```python
from build123d import *

# Parameters (mm, degrees)
BOSS_EXTRUDE1_DEPTH = 8
SKETCH2_R           = 5
BOSS_EXTRUDE2_DEPTH = 28
FILLET1_R           = 2
SKETCH3_R           = 1.55
CUT_EXTRUDE1_DEPTH  = 15.6
FILLET2_R           = 1
SKETCH5_R           = 2.1
CUT_EXTRUDE3_DEPTH  = 4
SKETCH6_R           = 0.5
CUT_EXTRUDE4_DEPTH  = 0.5
CUT_EXTRUDE5_REACH  = 10
SKETCH7_R           = 1


with BuildPart() as part:
    # Sketch1 → Boss-Extrude1 (new body)
    with BuildSketch(Plane(origin=(0, 0, 0), x_dir=(1, 0, 0), z_dir=(0, 1, 0))):
        Polygon((7.3, -4.214656965), (7.3, 4.214656965), (0, 8.42931393), (-7.3, 4.214656965), (-7.3, -4.214656965), (0, -8.42931393), align=None)
    extrude(amount=BOSS_EXTRUDE1_DEPTH)

    # Sketch2 → Boss-Extrude2 (add)
    with BuildSketch(Plane.XZ):
        Circle(SKETCH2_R)
        with BuildLine():
            Line((-1.55, 1.416862732), (-1.55, -1.416862732))
            ThreePointArc((-1.55, -1.416862732), (2.1, 0), (-1.55, 1.416862732))
        make_face(mode=Mode.SUBTRACT)
    extrude(amount=BOSS_EXTRUDE2_DEPTH)

    # Fillet1
    fillet1_edges = [part.edges().sort_by_distance(p)[0] for p in [
        (-5, 0, 0),
    ]]
    fillet(fillet1_edges, radius=FILLET1_R)

    # Sketch3 → Cut-Extrude1 (cut, through all)
    with BuildSketch(Plane(origin=(7.3, 0, 0), x_dir=(0, 0, -1), z_dir=(1, 0, 0))):
        with Locations((-0.085343035, 3.85)):
            Circle(SKETCH3_R)
    extrude(amount=-CUT_EXTRUDE1_DEPTH, mode=Mode.SUBTRACT)

    # Fillet2
    fillet2_edges = [part.edges().sort_by_distance(p)[0] for p in [
        (0, 4, 8.42931393),
        (-7.3, 4, 4.214656965),
        (-7.3, 4, -4.214656965),
        (0, 4, -8.42931393),
        (7.3, 4, -4.214656965),
        (7.3, 4, 4.214656965),
        (3.65, 8, -6.321985448),
        (-3.65, 8, -6.321985448),
        (-7.3, 8, 0),
        (-3.65, 8, 6.321985448),
        (3.65, 8, 6.321985448),
        (7.3, 8, 0),
    ]]
    fillet(fillet2_edges, radius=FILLET2_R)

    # Sketch5 → Cut-Extrude3 (cut)
    with BuildSketch(Plane.XZ.offset(28)):
        Circle(SKETCH5_R)
    extrude(amount=-CUT_EXTRUDE3_DEPTH, mode=Mode.SUBTRACT)

    # Sketch6 → Cut-Extrude4 (cut)
    with BuildSketch(Plane(origin=(3.65, 0, -6.321985448), x_dir=(-0.866025404, 0, -0.5), z_dir=(0.5, 0, -0.866025404))):
        with Locations((0, 3.5)):
            Circle(SKETCH6_R)
        with Locations((-2, 3.5)):
            Circle(SKETCH6_R)
        with Locations((2, 3.5)):
            Circle(SKETCH6_R)
    extrude(amount=-CUT_EXTRUDE4_DEPTH, mode=Mode.SUBTRACT)

    # Sketch7 → Cut-Extrude5 (cut, up to next)
    with BuildSketch(Plane.XZ, mode=Mode.PRIVATE) as cut_extrude5_sk1:
        Circle(SKETCH7_R)
    cut_extrude5_tool1 = extrude(cut_extrude5_sk1.sketch, amount=-CUT_EXTRUDE5_REACH, mode=Mode.PRIVATE) & part.part
    add(cut_extrude5_tool1.solids().sort_by_distance((0, 0, 0))[0], mode=Mode.SUBTRACT)


solid = part.part
```
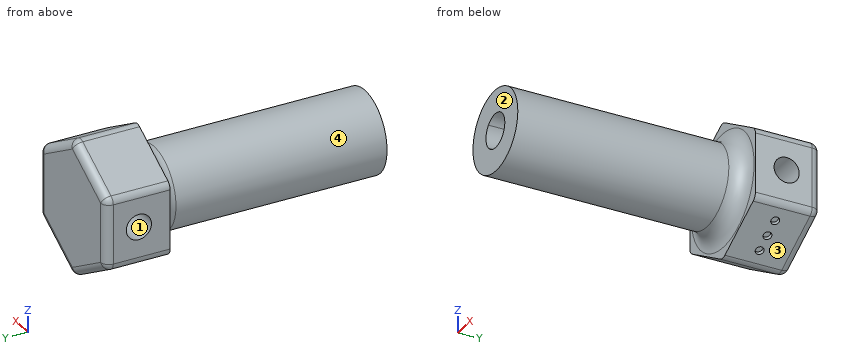
Check sheet for the modelled part. Datum: model origin and axes. Units: mm. Face numbers are marked on the shaded views. Round coordinates to 2 decimals unless told otherwise and drop trailing zeros. Loops run counter-clockwise (first coordinate to the right, second up) from the corner with the lowest first, then second, coordinate; pieces in that order, holes last. Notation, with made-up numbers: (13, 36.5) - (57, 36.5) arc R30 cw to (57, 63.5) - close; hole circle Ø3 at (34, 17). An arc over 180 degrees is marked (long way). Write item = value, one per line. Start each with the question number.
Q1. Section check D-D (y = -19). Record the boundary of the cut face in (x, z), plus the area to 3 significant figures.
Q2. Release check for a two-part mould opening along Z. For the marked faces 1, 2, 3 and 4 record: pulls with the +Z half, pulls with the -Z half, needs draft (parallel to the pull), parting line crosses it, or undercut.
Q3. Thickness scan on L1, parallel to X at y = 1.8, z = 0; L2, parallel to Z at x = 0, y = -13.5; L3, parallel to Y at x = 0, z = -1.25. Record the ranges inside material, lowest first.
Q4. Section check C-C (y = 1). Record the boundary of the cut face in (x, z), plus the area to 3 significant figures.
Q5. Depth check by flat-ended pin: P1, Ø1.5, axis at y = -18, z = 4, coming from the -X side; P2, Ø8, axis at x = 4.5, y = -21, coming from the +Z side; P3, Ø1, axis at x = -5.5, z = -3.5, coming from the -Y side; P4, Ø2.5, axis at y = 3.85, z = 0.09, coming from the -X side (3 decimals). Enter the tip coordinate at first touch or a pass-through.
Q6. Section check A-A (y = 5). Record the boundary of the cut face in (x, z).
Q7. Section check B-B (z = 0). Record the boundary of the cut face in (x, y).
Derived:
q1.outline = circle Ø10 at (0, 0); hole (-1.55, -1.42) arc R2.1 ccw (long way) to (-1.55, 1.42) - close
q1.area = 65.8 mm^2
q2.face_1 = undercut
q2.face_2 = needs draft
q2.face_3 = pulls with the -Z half
q2.face_4 = parting line crosses it
q3.L1 = -7.3 to -1, 1 to 7.3
q3.L2 = -5 to -2.1, 2.1 to 5
q3.L3 = 0 to 3.06, 4.64 to 8
q4.outline = (-7.3, -3.64) arc R1 ccw to (-6.8, -4.5) - (-0.5, -8.14) arc R1 ccw to (0.5, -8.14) - (6.8, -4.5) arc R1 ccw to (7.3, -3.64) - (7.3, 3.64) arc R1 ccw to (6.8, 4.5) - (0.5, 8.14) arc R1 ccw to (-0.5, 8.14) - (-6.8, 4.5) arc R1 ccw to (-7.3, 3.64) - close; hole circle Ø2 at (0, 0)
q4.area = 181 mm^2
q5.P1 = -3.8
q5.P2 = 4.97
q5.P3 = -0.26
q5.P4 = through
q6.outline = (-7.3, -3.64) arc R1 ccw to (-6.8, -4.5) - (-0.5, -8.14) arc R1 ccw to (0.5, -8.14) - (6.8, -4.5) arc R1 ccw to (7.3, -3.64) - (7.3, -0.95) - (-7.3, -0.95) - close; (-7.3, 1.12) - (7.3, 1.12) - (7.3, 3.64) arc R1 ccw to (6.8, 4.5) - (0.5, 8.14) arc R1 ccw to (-0.5, 8.14) - (-6.8, 4.5) arc R1 ccw to (-7.3, 3.64) - close
q7.outline = (-7.3, 0) - (-7, 0) arc R2 cw to (-5, -2) - (-5, -28) - (-2.1, -28) - (-2.1, -24) - (-1.55, -24) - (-1.55, 0) - (-1, 0) - (-1, 2.3) - (-7.3, 2.3) - close; (-7.3, 5.4) - (7.3, 5.4) - (7.3, 7) arc R1 ccw to (6.3, 8) - (-6.3, 8) arc R1 ccw to (-7.3, 7) - close; (1, 0) - (2.1, 0) - (2.1, -28) - (5, -28) - (5, -2) arc R2 cw to (7, 0) - (7.3, 0) - (7.3, 2.3) - (1, 2.3) - close
